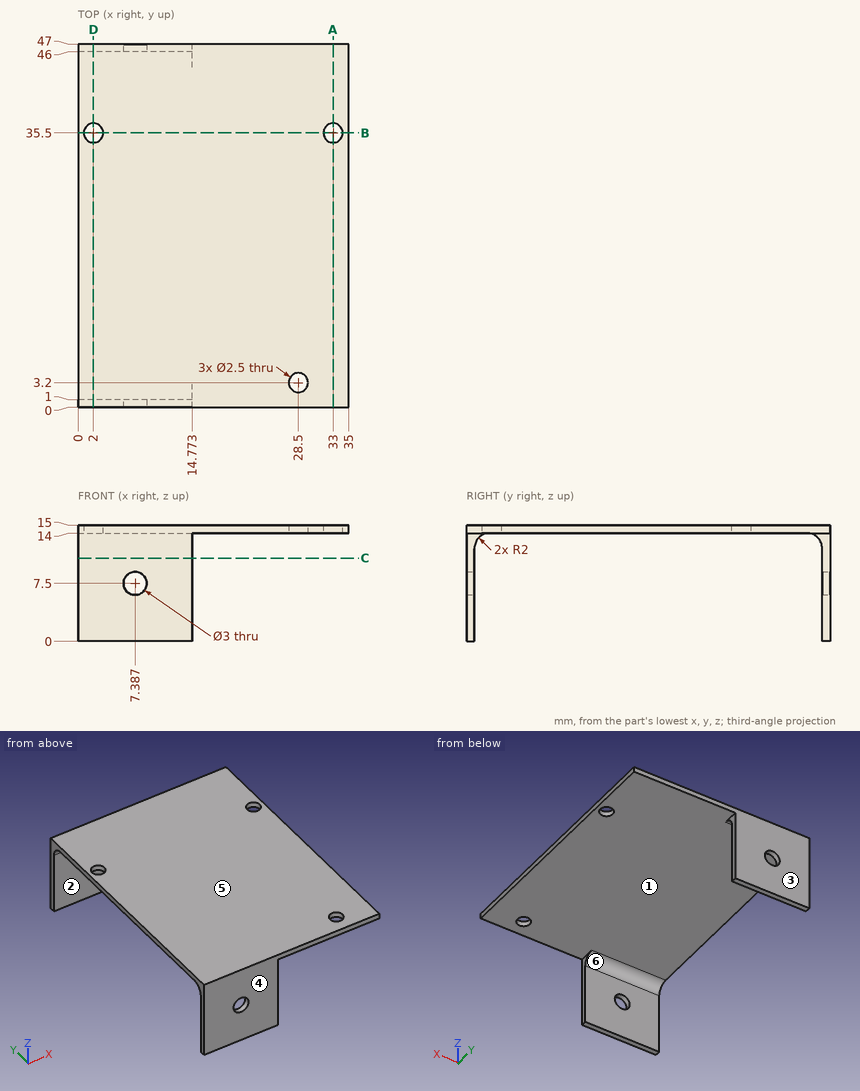
Print and shaded views of the part. All mm, measured from the part's lowest x, y and z. A direction names the side the tool comes from. Round coordinates to 2 decimals unless told otherwise and drop trailing zeros. Write each loop counter-clockwise with the first axis right and the second up, starting at its lowest first coordinate (ties: lowest second). Pieces come first, ordered by that corner, then holes. Notation, with made-up numbers: (76.25, 32) - (86.25, 32) arc R28 cw to (86.25, 52) - close; hole circle Ø2 at (47.25, 83). An arc over 180 degrees is marked (long way). One line per question, with ' | ' between items.
1. Band-saw the part on D-D, the plane x = 2. Write the cut outline in (y, z).
Results are:
outline: (0, 0) - (1, 0) - (1, 12) arc R2 cw to (3, 14) - (34.25, 14) - (34.25, 15) - (0, 15) - close; (36.75, 14) - (44, 14) arc R2 cw to (46, 12) - (46, 0) - (47, 0) - (47, 15) - (36.75, 15) - close
2. Band-saw the part on C-C, the plane z = 10.75. Write the cut outline in (x, y).
Results are:
outline: (0, 0) - (14.77, 0) - (14.77, 1) - (0, 1) - close; (0, 46) - (14.77, 46) - (14.77, 47) - (0, 47) - close
3. Mould opens along Y. For the marked faces 1, 2, 3 and 4 say: released by +Y, released by -Y, zero draft, split by the parting line, or undercut.
Results are:
face 1: undercut | face 2: undercut | face 3: released by +Y | face 4: released by -Y
4. Drill centre lines: line 1 along Y through (x, z) = (28.5, 14.8); line 2 along Y through (x, z) = (4, 8.5); line 3 along Z through (x, y) = (14.5, 19). Where is each one in solid material? Low to high. Write a range as from..to.
Results are:
line 1: 0..1.95, 4.45..47 | line 2: 0..1, 46..47 | line 3: 14..15
5. Band-saw the part on B-B, the plane y = 35.5. Write the cut outline in (x, z).
Results are:
outline: (0, 14) - (0.75, 14) - (0.75, 15) - (0, 15) - close; (3.25, 14) - (31.75, 14) - (31.75, 15) - (3.25, 15) - close; (34.25, 14) - (35, 14) - (35, 15) - (34.25, 15) - close
6. Tool access for the marked faces 5 and 6: list every direction of +Z, -Z, +X, -X, +Y, -Y with a clear straight run to the whole face (end or side of a thin tool).
Results are:
face 5: +Z, +X, -X, +Y, -Y | face 6: -Z, +X, -X
7. Band-saw the part on A-A, the plane x = 33. Write the cut outline in (y, z).
Results are:
outline: (0, 14) - (34.25, 14) - (34.25, 15) - (0, 15) - close; (36.75, 14) - (47, 14) - (47, 15) - (36.75, 15) - close
8. Drop flat-ended pins along their axis: pin 1 Ø2 at (x, z) = (29.5, 11.5) entering from -Y; pin 2 Ø3.5 at (y, z) = (46, 5) entering from +X. Give the stop position or say it passes through.
Results are:
pin 1: through | pin 2: x = 14.77
